Input: part model. Units: mm. Frame: model coordinates. A direction names the side the tool comes from. Coordinates: 2 decimals unless noted, no trailing zeros. Order: outer loops, then holes, each group sorted by start corner. A loop starts at its lowest first (then second) coordinate and runs counter-clockwise, first axis right, second up. Notation, with made-up numbers: M 83,-39 L 114,-39 A29 ccw 114,0 Z; hole C -38.5,-14.75 d1. An arc over 180 degrees is marked long. One line per item, written item: value.
```python
from build123d import *


with BuildPart() as part:
    # Esquisse1 → Révolution1 (revolve)
    with BuildSketch(Plane(origin=(0, 0, 0), x_dir=(0, 0, -1), z_dir=(1, 0, 0))):
        with BuildLine():
            Line((8, -5), (8, 0))
            Line((8, 0), (6, 0))
            Line((6, 0), (6, 12))
            Line((6, 12), (0, 12))
            Line((0, 12), (0, -50))
            Line((0, -50), (23.580737766, -50))
            ThreePointArc((23.580737766, -50), (24.957446917, -49.450748742), (25.577996835, -48.104671912))
            Line((25.577996835, -48.104671912), (25.99725907, -40.104671912))
            ThreePointArc((25.99725907, -40.104671912), (25.554291923, -38.741359218), (24.31286893, -38.024623319))
            Line((24.31286893, -38.024623319), (22.923403705, -37.804553647))
            ThreePointArc((22.923403705, -37.804553647), (20.696139769, -36.657437342), (19.58806929, -34.410492688))
            Line((19.58806929, -34.410492688), (15.938619423, -8.443307596))
            ThreePointArc((15.938619423, -8.443307596), (14.601783264, -5.981161679), (11.977547148, -5))
            Line((11.977547148, -5), (8, -5))
        make_face()
    revolve(axis=Axis((0, 12, 0), (0, -1, 0)))


solid = part.part
```
(1) First-contact query: pin 1 (12 mm diameter, centred on y = -38, z = -1.5, fed in from -X); pin 2 (8 mm diameter, centred on y = -12, z = -3.5, fed in from -X); pin 3 (1.5 mm diameter, centred on x = 11, z = 7, fed in from +Y). Flat tips, straight axial feed; report the tip coordinate or a pass-through.
Data:
pin 1: stops at x = -26
pin 2: stops at x = -16.86
pin 3: stops at y = -5.01
(2) Cut plane D-D on y = 6.5. Output: boundary loops of the cut face in (x, z).
Data:
outline: C 0,0 d12
(3) Cut plane A-A on x = 0. Output: boundary loops of the cut face in (y, z), plus the area to 3 significant figures.
Data:
outline: M -50,-23.58 A2 ccw -48.1,-25.58 L -40.1,-26 A2 ccw -38.02,-24.31 L -37.8,-22.92 A4 cw -34.41,-19.59 L -8.44,-15.94 A4 ccw -5,-11.98 L -5,-8 L 0,-8 L 0,-6 L 12,-6 L 12,6 L 0,6 L 0,8 L -5,8 L -5,11.98 A4 ccw -8.44,15.94 L -34.41,19.59 A4 cw -37.8,22.92 L -38.02,24.31 A2 ccw -40.1,26 L -48.1,25.58 A2 ccw -50,23.58 Z
area: 2,010 mm2
(4) Cut plane B-B on z = 0. Output: boundary loops of the cut face in (x, y).
Data:
outline: M -26,-40.1 L -25.58,-48.1 A2 ccw -23.58,-50 L 23.58,-50 A2 ccw 25.58,-48.1 L 26,-40.1 A2 ccw 24.31,-38.02 L 22.92,-37.8 A4 cw 19.59,-34.41 L 15.94,-8.44 A4 ccw 11.98,-5 L 8,-5 L 8,0 L 6,0 L 6,12 L -6,12 L -6,0 L -8,0 L -8,-5 L -11.98,-5 A4 ccw -15.94,-8.44 L -19.59,-34.41 A4 cw -22.92,-37.8 L -24.31,-38.02 A2 ccw Z
(5) Cut plane C-C on y = -16.5. Output: boundary loops of the cut face in (x, z), plus the area to 3 significant figures.
Data:
outline: C 0,0 d34.14
area: 916 mm2
(6) Access query for faces 1 (the flat face through (0, 12, 0)), 2 (the cylindrical face through (-7.81, -2.46, 1.73)). Directions: +Z, -Z, +X, -X, +Y, -Y. A direction counts if a zero-diameter tool reaches every point of the face in a straight line with its end or side. Return the directions, or none.
Data:
face 1: +Z, -Z, +X, -X, +Y
face 2: +Y
(7) Ray query, line 1 (X direction, y = -28, z = 8); line 2 (Y direction, x = -5, z = -20.5); line 3 (Y direction, x = -5, z = 21). Return the intervals inside material, ascending. Write a range as from..to.
Data:
line 1: x = -16.89..16.89
line 2: y = -50..-37.02
line 3: y = -50..-37.34
